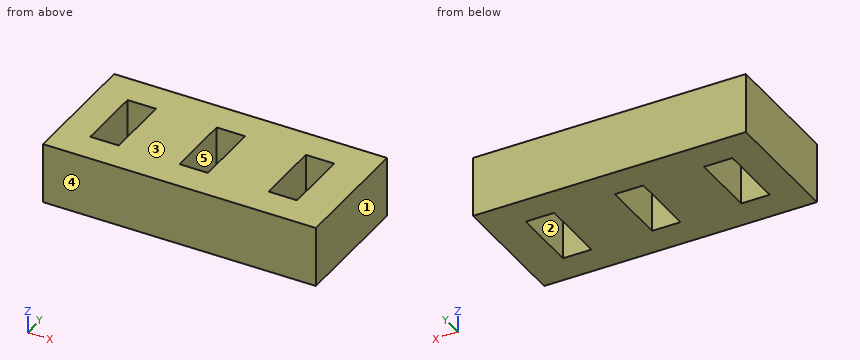
```python
from build123d import *

# Parameters (mm, degrees)
BOX_W        = 4.7
BOX_H        = 11
BOX_DEPTH    = 13
BOX001_W     = 4.7
BOX001_H     = 11
BOX001_DEPTH = 13
BOX002_W     = 4.7
BOX002_H     = 11
BOX002_DEPTH = 13
BOX003_W     = 45
BOX003_H     = 21
BOX003_DEPTH = 10


with BuildPart() as cub:
    # Box → Box (new body)
    with BuildSketch(Plane.XY.offset(-1)):
        with Locations((2.35, 5.5)):
            Rectangle(BOX_W, BOX_H)
    extrude(amount=BOX_DEPTH)


with BuildPart() as cub001:
    # Box001 → Box001 (new body)
    with BuildSketch(Plane(origin=(14.7, 0, -1), x_dir=(1, 0, 0), z_dir=(0, 0, 1))):
        with Locations((2.35, 5.5)):
            Rectangle(BOX001_W, BOX001_H)
    extrude(amount=BOX001_DEPTH)


with BuildPart() as cub002:
    # Box002 → Box002 (new body)
    with BuildSketch(Plane(origin=(29.4, 0, -1), x_dir=(1, 0, 0), z_dir=(0, 0, 1))):
        with Locations((2.35, 5.5)):
            Rectangle(BOX002_W, BOX002_H)
    extrude(amount=BOX002_DEPTH)


with BuildPart() as cut002:
    # Box003 → Box003 (new body)
    with BuildSketch(Plane(origin=(-5, -5, 0), x_dir=(1, 0, 0), z_dir=(0, 0, 1))):
        with Locations((22.5, 10.5)):
            Rectangle(BOX003_W, BOX003_H)
    extrude(amount=BOX003_DEPTH)

    # Cut: cut Cub002
    add(cub002.part, mode=Mode.SUBTRACT)

    # Cut001: cut Cub001
    add(cub001.part, mode=Mode.SUBTRACT)

    # Cut002: cut Cub
    add(cub.part, mode=Mode.SUBTRACT)


solid = cut002.part
```
Build history of the part. All positions in model axes, mm. Face numbers are marked on the shaded views. A direction names the side the tool comes from. Give positions to 0.01 mm unless a question says otherwise; leave off trailing zeros. Order: outer loops, then holes, each group sorted by start corner. A loop starts at its lowest first (then second) coordinate and runs counter-clockwise, first axis right, second up. Notation, with made-up numbers: M -28.75,82.5 L -12.75,82.5 A12 ccw -12.75,97.5 Z; hole C 80.25,83 d10. An arc over 180 degrees is marked long. Write item = value, one per line. Start each with the question number.
(1) Slice it at B-B on z = 7.75. Write the cut outline in (x, y).
(2) Probe L1, parallel to X at y = 4.25, z = 6; L2, parallel to Y at x = 17, z = 1.5. List the from-to ranges inside material, lowest first. Write a range as [from, to].
(3) Which spindle directions (+Z, -Z, +X, -X, +Y, -Y) get a long thin tool onto all of the face, cutting with end or side? Do the marked faces 4 and 5. Say none if no direction does.
(4) Slice it at A-A on y = 2.25. Write the cut outline in (x, z).
(5) Two-plate mould, pull along X, no slides. Class the marked faces 1, 2 and 3: released by +X, released by -X, zero draft, split by the parting line, or undercut.
Responses:
q1.outline = M -5,-5 L 40,-5 L 40,16 L -5,16 Z; hole M 0,0 L 4.7,0 L 4.7,11 L 0,11 Z; hole M 14.7,0 L 19.4,0 L 19.4,11 L 14.7,11 Z; hole M 29.4,0 L 34.1,0 L 34.1,11 L 29.4,11 Z
q2.L1 = [-5, 0], [4.7, 14.7], [19.4, 29.4], [34.1, 40]
q2.L2 = [-5, 0], [11, 16]
q3.face_4 = +Z, -Z, +X, -X, -Y
q3.face_5 = +Z, -Z
q4.outline = M -5,0 L 0,0 L 0,10 L -5,10 Z; M 4.7,0 L 14.7,0 L 14.7,10 L 4.7,10 Z; M 19.4,0 L 29.4,0 L 29.4,10 L 19.4,10 Z; M 34.1,0 L 40,0 L 40,10 L 34.1,10 Z
q5.face_1 = released by +X
q5.face_2 = undercut
q5.face_3 = zero draft
